Source: CAD feature listing. Evaluate the final solid. Frame: model axes, mm. Face numbers are marked on the shaded views. A direction names the side the tool comes from. Round coordinates to 2 decimals unless told otherwise and drop trailing zeros. Write each loop counter-clockwise with the first axis right and the second up, starting at its lowest first coordinate (ties: lowest second). Pieces come first, ordered by that corner, then holes.
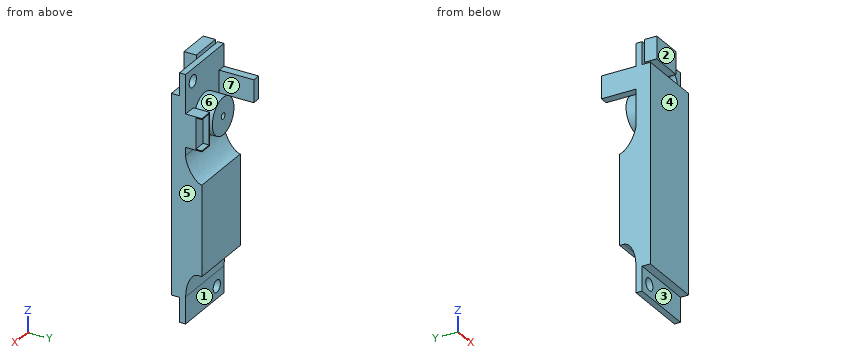
```python
from build123d import *

# Parameters (mm, degrees)
SKETCH1_W           = 16
SKETCH1_H           = 60
BOSS_EXTRUDE1_DEPTH = 1.5
SKETCH5_R           = 1.5
CUT_EXTRUDE1_DEPTH  = 32.084562085
SKETCH8_W           = 16
SKETCH8_H           = 22
BOSS_EXTRUDE2_DEPTH = 4
FILLET1_START       = -8
FILLET1_DEPTH       = 16
FILLET2_START       = -8
FILLET2_DEPTH       = 16
SKETCH12_W          = 3.25
SKETCH12_H          = 8
BOSS_EXTRUDE5_DEPTH = 4
SKETCH15_R          = 4.5
BOSS_EXTRUDE6_DEPTH = 4.5
SKETCH16_W          = 3
SKETCH16_H          = 7.5
CUT_EXTRUDE2_DEPTH  = 1.5
SKETCH17_R          = 0.75
CUT_EXTRUDE3_DEPTH  = 1
SKETCH18_W          = 2
SKETCH18_H          = 5.5
BOSS_EXTRUDE7_DEPTH = 8.5
SKETCH22_W          = 8
SKETCH22_H          = 5.5
BOSS_EXTRUDE8_DEPTH = 3
SKETCH23_W          = 16
SKETCH23_H          = 48.5
BOSS_EXTRUDE9_DEPTH = 2


with BuildPart() as part:
    # Sketch1 → Boss-Extrude1 (new body)
    with BuildSketch(Plane(origin=(0, 0, 0), x_dir=(1, 0, 0), z_dir=(0, 1, 0))):
        Rectangle(SKETCH1_W, SKETCH1_H)
    extrude(amount=BOSS_EXTRUDE1_DEPTH)

    # Sketch5 → Cut-Extrude1 (cut, through all)
    with BuildSketch(Plane(origin=(0, 1.5, 0), x_dir=(1, 0, 0), z_dir=(0, 1, 0))):
        with Locations(Location((-5, 27, 0), (0, 0, 270))):
            Circle(SKETCH5_R)
        with Locations(Location((5, -27, 0), (0, 0, 270))):
            Circle(SKETCH5_R)
    extrude(amount=-CUT_EXTRUDE1_DEPTH, mode=Mode.SUBTRACT)

    # Sketch8 → Boss-Extrude2 (add)
    with BuildSketch(Plane(origin=(0, 1.5, 0), x_dir=(1, 0, 0), z_dir=(0, 1, 0))):
        with Locations((0, 6.5)):
            Rectangle(SKETCH8_W, SKETCH8_H)
    extrude(amount=BOSS_EXTRUDE2_DEPTH)

    # Fillet1: read off the stored shape, not the designer's step
    # Fillet1 outline → Fillet1 (add)
    with BuildSketch(Plane.YZ.offset(FILLET1_START)):
        with BuildLine():
            Line((1.5, -17.5), (1.5, -23.5))
            add(Edge.make_bspline(
                [(1.5, -23.5), (1.5, -17.5), (4.5, -17.5)],
                knots=[0, 0, 0, 1, 1, 1], degree=2, weights=[1, 0.666666667, 1]))
            Line((4.5, -17.5), (1.5, -17.5))
        make_face()
    extrude(amount=FILLET1_DEPTH)

    # Fillet2: read off the stored shape, not the designer's step
    # Fillet2 outline → Fillet2 (add)
    with BuildSketch(Plane.YZ.offset(FILLET2_START)):
        with BuildLine():
            Line((1.5, 4.5), (5.5, 4.5))
            add(Edge.make_bspline(
                [(5.5, 4.5), (1.5, 4.5), (1.5, 10.5)],
                knots=[0, 0, 0, 1, 1, 1], degree=2, weights=[1, 0.428571429, 1]))
            Line((1.5, 10.5), (1.5, 4.5))
        make_face()
    extrude(amount=FILLET2_DEPTH)

    # Sketch12 → Boss-Extrude5 (add)
    with BuildSketch(Plane(origin=(0, 1.5, 0), x_dir=(1, 0, 0), z_dir=(0, 1, 0))):
        with Locations((6.375, -16.5)):
            Rectangle(SKETCH12_W, SKETCH12_H)
    extrude(amount=BOSS_EXTRUDE5_DEPTH)

    # Sketch15 → Boss-Extrude6 (add)
    with BuildSketch(Plane(origin=(0, 1.5, 0), x_dir=(1, 0, 0), z_dir=(0, 1, 0))):
        with Locations(Location((0, -17.5, 0), (0, 0, 270))):
            Circle(SKETCH15_R)
    extrude(amount=BOSS_EXTRUDE6_DEPTH)

    # Sketch16 → Cut-Extrude2 (cut)
    with BuildSketch(Plane(origin=(0, 5.5, 0), x_dir=(1, 0, 0), z_dir=(0, 1, 0))):
        with Locations((6.5, -16.5)):
            Rectangle(SKETCH16_W, SKETCH16_H)
    extrude(amount=-CUT_EXTRUDE2_DEPTH, mode=Mode.SUBTRACT)

    # Sketch17 → Cut-Extrude3 (cut)
    with BuildSketch(Plane(origin=(0, 6, 0), x_dir=(1, 0, 0), z_dir=(0, 1, 0))):
        with Locations(Location((0, -17.5, 0), (0, 0, 270))):
            Circle(SKETCH17_R)
    extrude(amount=-CUT_EXTRUDE3_DEPTH, mode=Mode.SUBTRACT)

    # Sketch18 → Boss-Extrude7 (add)
    with BuildSketch(Plane(origin=(0, 1.5, 0), x_dir=(1, 0, 0), z_dir=(0, 1, 0))):
        with Locations((-7, -21.75)):
            Rectangle(SKETCH18_W, SKETCH18_H)
    extrude(amount=BOSS_EXTRUDE7_DEPTH)

    # Sketch22 → Boss-Extrude8 (add)
    with BuildSketch(Plane.XZ):
        with Locations((-3, 28.25)):
            Rectangle(SKETCH22_W, SKETCH22_H)
    extrude(amount=BOSS_EXTRUDE8_DEPTH)

    # Sketch23 → Boss-Extrude9 (add)
    with BuildSketch(Plane.XZ):
        with Locations((0, 0.25)):
            Rectangle(SKETCH23_W, SKETCH23_H)
    extrude(amount=BOSS_EXTRUDE9_DEPTH)


solid = part.part
```
Q1. Pin query (flat end, axial travel): P1, Ø0.8, axis at x = 6.5, y = 5, coming from the -Z side; P2, Ø2.5, axis at x = -5, z = -27, coming from the -Y side; P3, Ø1.6, axis at x = -3.5, y = 1, coming from the +Z side; P4, Ø2.5, axis at x = -2, y = -1.5, coming from the -Z side. Return the tip coordinate at first contact, or that it passes through.
Q2. Section query B-B, the plane y = -0.75. Output: boundary loops of the cut face in (x, z).
Q3. Set-up query: the marked faces 1, 2 and 3. Return all of +Z, -Z, +X, -X, +Y, -Y with unobstructed straight access to the full face (end or side cutting, diameter ignored); none if empty.
Q4. Section query C-C, the plane z = -27. Output: boundary loops of the cut face in (x, y), and give its area (3 significant figures).
Q5. Section query D-D, the plane z = 1.5. Output: boundary loops of the cut face in (x, y), and give its area (3 significant figures).
Q6. Line query: line 1 (X direction, y = 0.9, z = -27); line 2 (Z direction, x = 6, y = 5); line 3 (X direction, y = 0.9, z = 27). Output: solid intervals per line, ascending.
Q7. Mould query, pull axis X, two halves, no side actions, for the marked faces 4, 5, 6 and 7. Classes: pulls with the +X half, pulls with the -X half, needs draft (parallel to the pull), parting line crosses it, or undercut.
Q8. Section query A-A, the plane z = 27. Output: boundary loops of the cut face in (x, y), and give its area (3 significant figures).
Filled in:
1. P1: stops at z = -17.5
1. P2: passes through
1. P3: stops at z = 30
1. P4: stops at z = -24
2. outline: (-8, -24) - (8, -24) - (8, 24.5) - (-8, 24.5) - close; (-7, 25.5) - (1, 25.5) - (1, 31) - (-7, 31) - close
3. face 1: -Z, +X, -X, +Y
3. face 2: +Z, -Z, +X, -X, -Y
3. face 3: -Z, +X, -X, -Y
4. outline: (-8, 0) - (-6.5, 0) - (-6.5, 1.5) - (-8, 1.5) - close; (-3.5, 0) - (8, 0) - (8, 1.5) - (-3.5, 1.5) - close
4. area: 19.5 mm2
5. outline: (-8, -2) - (8, -2) - (8, 5.5) - (-8, 5.5) - close
5. area: 120 mm2
6. line 1: x = -8 to -6.5, -3.5 to 8
6. line 2: z = -17.5 to 4.61, 12.5 to 12.75, 20.25 to 20.5
6. line 3: x = -8 to 3.5, 6.5 to 8
7. face 4: needs draft
7. face 5: pulls with the +X half
7. face 6: undercut
7. face 7: undercut
8. outline: (-8, 0) - (-7, 0) - (-7, -3) - (1, -3) - (1, 0) - (3.5, 0) - (3.5, 1.5) - (-8, 1.5) - close; (6.5, 0) - (8, 0) - (8, 1.5) - (6.5, 1.5) - close
8. area: 43.5 mm2
